Could you check a few things on this model? Use its own coordinates, in mm. Face numbers are marked on the shaded views. A direction names the side the tool comes from. Coordinates: 2 decimals unless noted, no trailing zeros. Loops run counter-clockwise (first coordinate to the right, second up) from the corner with the lowest first, then second, coordinate; pieces in that order, holes last.
1) Will these pins go through, and if not, where does the flat tip stop? P1, Ø6, axis at y = 6.5, z = -22, coming from the -X side; P2, Ø2.5, axis at x = 0, z = 0, coming from the -Y side; P3, Ø4, axis at x = -0.5, z = -20, coming from the -Y side; P4, Ø3, axis at x = 4.5, y = -3.5, coming from the +Z side.
2) Imagine slicing it at C-C on x = 1. Please give me the cut outline in (y, z).
3) Imagine slicing it at D-D on y = 5.5. Please give me the cut outline in (x, z).
4) If I drill on line 1 along X through (y, z) = (3.75, -16.5); line 2 along Z through (x, y) = (0, 4); line 3 along Z through (x, y) = (0, 8.5), over which ranges is the centre line in solid material (lowest first)?
5) For the marked faces 1 and 2, which set-ups out of +Z, -Z, +X, -X, +Y, -Y let a thin tool reach every point of the face, with its end or its side?
6) Imagine slicing it at B-B on x = 6.25. Please give me the cut outline in (y, z), plus the area to 3 significant figures.
7) Imagine slicing it at A-A on y = 9. Please give me the cut outline in (x, z), plus the area to 3 significant figures.
```python
from build123d import *

# Parameters (mm, degrees)
SKETCH1_W                = 7
SKETCH1_H                = 16
SKETCH1_W_2              = 3.5
BOSS_EXTRUDE1_DEPTH      = 14.2
M3_CLEARANCE_HOLE1_D     = 3.2
M5_CLEARANCE_HOLE1_D     = 5.3
SKETCH6_W                = 14.632471907
SKETCH6_H                = 4
BOSS_EXTRUDE2_DEPTH      = 6
BOSS_EXTRUDE2_DEPTH_BACK = 14.2
FILLET1_R                = 1
FILLET2_R                = 2
SKETCH7_W                = 8.569742994
SKETCH7_H                = 13.514047563
CUT_EXTRUDE1_DEPTH       = 10
CHAMFER1_SIZE            = 13
FILLET4_R                = 2


with BuildPart() as part:
    # Sketch1 → Boss-Extrude1 (new body)
    with BuildSketch(Plane(origin=(0, 0, 0), x_dir=(1, 0, 0), z_dir=(0, 1, 0))):
        with BuildLine():
            Line((-3.5, 16.5), (3.5, 16.5))
            ThreePointArc((3.5, 16.5), (3.498391173, 16.393890619), (3.493566171, 16.287878788))
            Line((3.493566171, 16.287878788), (2.495404408, -0.151515152))
            ThreePointArc((2.495404408, -0.151515152), (0, -2.5), (-2.495404408, -0.151515152))
            Line((-2.495404408, -0.151515152), (-3.493566171, 16.287878788))
            ThreePointArc((-3.493566171, 16.287878788), (-3.498391173, 16.393890619), (-3.5, 16.5))
        make_face()
        with Locations((0, 24.5)):
            Rectangle(SKETCH1_W, SKETCH1_H)
        with BuildLine():
            ThreePointArc((2.495404408, -0.151515152), (1.713361042, -1.820547703), (0, -2.5))
            Line((0, -2.5), (9, -2.5))
            Line((9, -2.5), (9, 32.5))
            Line((9, 32.5), (3.5, 32.5))
            Line((3.5, 32.5), (3.5, 16.5))
            ThreePointArc((3.5, 16.5), (3.498391173, 16.393890619), (3.493566171, 16.287878788))
            Line((3.493566171, 16.287878788), (2.495404408, -0.151515152))
        make_face()
        with BuildLine():
            Line((0, 16.5), (0, -2.5))
            ThreePointArc((0, -2.5), (1.713361042, -1.820547703), (2.495404408, -0.151515152))
            Line((2.495404408, -0.151515152), (3.493566171, 16.287878788))
            ThreePointArc((3.493566171, 16.287878788), (3.498391173, 16.393890619), (3.5, 16.5))
            Line((3.5, 16.5), (0, 16.5))
        make_face()
        with Locations((1.75, 24.5)):
            Rectangle(SKETCH1_W_2, SKETCH1_H)
    extrude(amount=BOSS_EXTRUDE1_DEPTH)

    # M3 Clearance Hole1 (through all)
    with Locations(Plane(origin=(0, 0, 0), x_dir=(-1, 0, 0), z_dir=(0, -1, 0))):
        with Locations((0, 0)):
            Hole(M3_CLEARANCE_HOLE1_D / 2)

    # M5 Clearance Hole1 (through all)
    with Locations(Plane(origin=(0, 0, 0), x_dir=(-1, 0, 0), z_dir=(0, -1, 0))):
        with Locations((0, 16.5)):
            Hole(M5_CLEARANCE_HOLE1_D / 2)

    # Sketch6 → Boss-Extrude2 (add, two sides)
    with BuildSketch(Plane.XZ) as boss_extrude2_sk:
        with Locations((1.683764046, -34.5)):
            Rectangle(SKETCH6_W, SKETCH6_H)
    extrude(amount=BOSS_EXTRUDE2_DEPTH)
    extrude(boss_extrude2_sk.sketch, amount=-BOSS_EXTRUDE2_DEPTH_BACK)

    # Fillet1
    fillet1_edges = [part.edges().sort_by_distance(p)[0] for p in [
        (2.75, 0, -32.5),
    ]]
    fillet(fillet1_edges, radius=FILLET1_R)

    # Fillet2
    fillet2_edges = [part.edges().sort_by_distance(p)[0] for p in [
        (9, 7.1, 2.5),
    ]]
    fillet(fillet2_edges, radius=FILLET2_R)

    # Sketch7 → Cut-Extrude1 (cut)
    with BuildSketch(Plane.XZ):
        with Locations((-7.784871497, -36.46322787)):
            Rectangle(SKETCH7_W, SKETCH7_H)
    extrude(amount=-CUT_EXTRUDE1_DEPTH, mode=Mode.SUBTRACT)

    # Chamfer1
    chamfer1_edges = [part.edges().sort_by_distance(p)[0] for p in [
        (1.683764046, 14.2, -36.5),
    ]]
    chamfer(chamfer1_edges, length=CHAMFER1_SIZE)

    # Fillet4
    fillet4_edges = [part.edges().sort_by_distance(p)[0] for p in [
        (2.75, 1.2, -36.5),
        (2.75, 14.2, -23.5),
    ]]
    fillet(fillet4_edges, radius=FILLET4_R)


solid = part.part
```
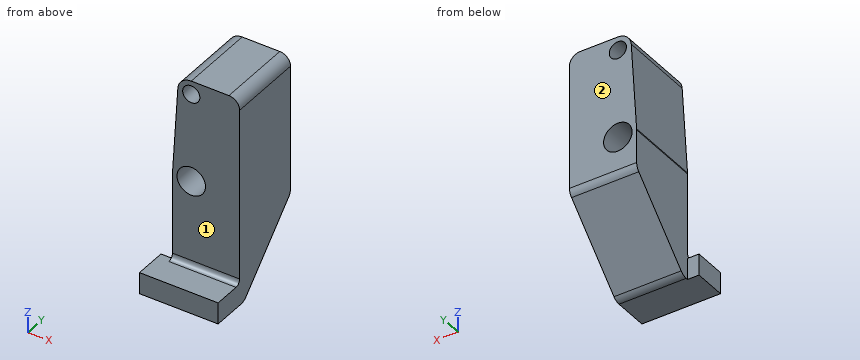
Filled in:
1. P1: stops at x = -3.5
1. P2: passes through
1. P3: stops at y = 0
1. P4: stops at z = -32.5
2. outline: (-6, -36.5) - (0.37, -36.5) arc R2 ccw to (1.79, -35.91) - (13.61, -24.09) arc R2 ccw to (14.2, -22.67) - (14.2, -18.95) - (0, -18.95) - (0, -31.5) arc R1 cw to (-1, -32.5) - (-6, -32.5) - close; (0, -14.05) - (14.2, -14.05) - (14.2, -1.25) - (0, -1.25) - close; (0, 1.25) - (14.2, 1.25) - (14.2, 2.5) - (0, 2.5) - close
3. outline: (-3.5, -32.2) - (9, -32.2) - (9, 0.5) arc R2 ccw to (7, 2.5) - (0, 2.5) arc R2.5 ccw to (-2.5, 0.15) - (-3.49, -16.29) arc R3.5 ccw to (-3.5, -16.5) - close; hole circle Ø5.3 at (0, -16.5); hole circle Ø3.2 at (0, 0)
4. line 1: x = -3.5 to -2.65, 2.65 to 9
4. line 2: z = -33.7 to -19.15, -13.85 to -1.6, 1.6 to 2.5
4. line 3: z = -29.2 to -19.15, -13.85 to -1.6, 1.6 to 2.5
5. face 1: +Z, +X, -X, -Y
5. face 2: +Z, -Z, +X, -X, +Y
6. outline: (-6, -36.5) - (0.37, -36.5) arc R2 ccw to (1.79, -35.91) - (13.61, -24.09) arc R2 ccw to (14.2, -22.67) - (14.2, 2.5) - (0, 2.5) - (0, -31.5) arc R1 cw to (-1, -32.5) - (-6, -32.5) - close
6. area: 493 mm2
7. outline: (-3.5, -28.7) - (9, -28.7) - (9, 0.5) arc R2 ccw to (7, 2.5) - (0, 2.5) arc R2.5 ccw to (-2.5, 0.15) - (-3.49, -16.29) arc R3.5 ccw to (-3.5, -16.5) - close; hole circle Ø5.3 at (0, -16.5); hole circle Ø3.2 at (0, 0)
7. area: 347 mm2
